The drawing under review shows one solid part. Ordinate dimensions are in mm from its lowest x, y, z. A direction names the side the tool comes from. Round coordinates to 2 decimals unless told otherwise and drop trailing zeros. Order: outer loops, then holes, each group sorted by start corner. A loop starts at its lowest first (then second) coordinate and runs counter-clockwise, first axis right, second up.
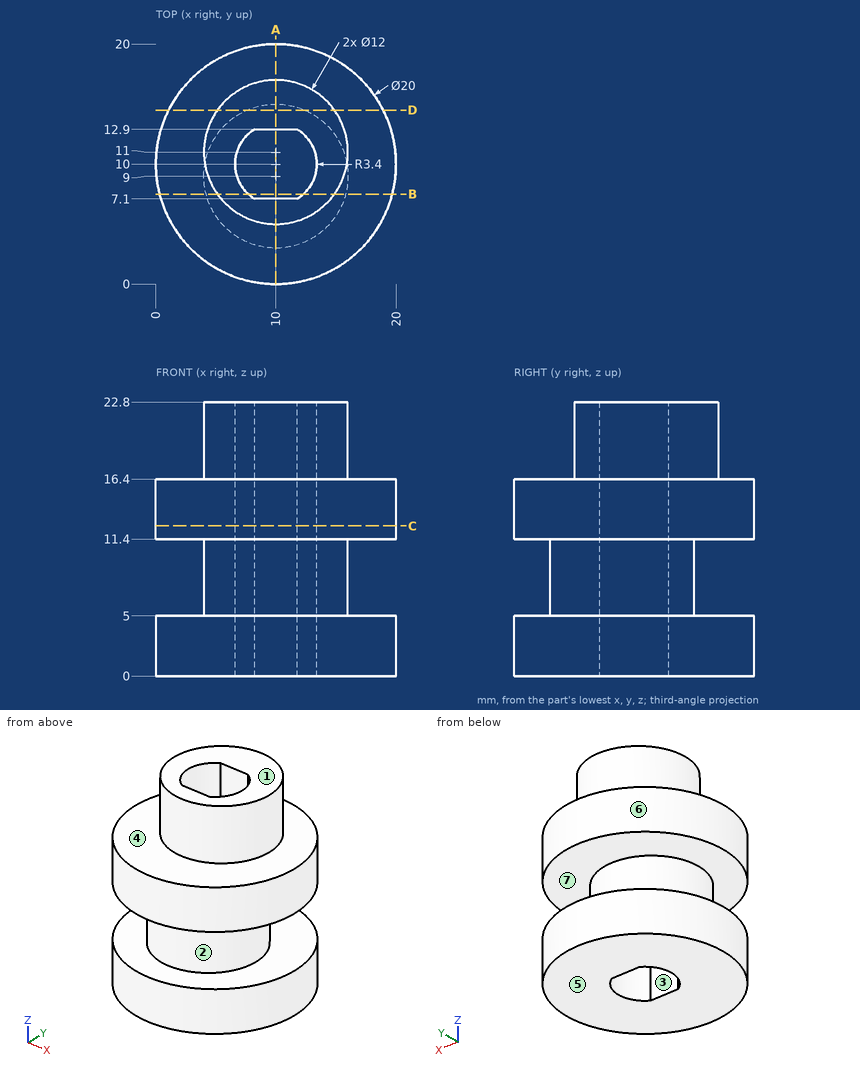
Q1. Tool access review of the marked faces 1, 2, 3 and 4: name each direction out of +Z, -Z, +X, -X, +Y, -Y from which nothing blocks a thin tool from reaching the whole face with its end or side.
Q2. Take a section at B-B, the plane y = 7.5. State the section outline as (x, z) points, plus the area to 3 significant figures.
Q3. Mouldability with a two-part tool opening along Z and no side actions: class the marked faces 5, 6 and 7 as +Z half, -Z half, draft (parallel to the pull), parting line (faces both ways), or undercut.
Q4. Take a section at C-C, the plane z = 12.5. State the section outline as (x, y) points.
Q5. Take a section at A-A, the plane x = 10. State the section outline as (y, z) points, plus the area to 3 significant figures.
Q6. Clearance check with flat-ended pins moving along their axes: pin 1 (1.5 mm diameter, centred on x = 8, y = 8.5, fed in from -Z); pin 2 (1.5 mm diameter, centred on x = 3.5, z = 15, fed in from +Y); pin 3 (1.5 mm diameter, centred on x = 17, y = 14.5, fed in from +Z); pin 4 (3 mm diameter, centred on x = 7, z = 7, fed in from +Y). State where each tip first meets the part, or that it passes through.
Q7. Take a section at D-D, the plane y = 14.5. State the section outline as (x, z) points.
Q8. Wall thickness on line 1 (Z direction, x = 5.5, y = 18.5); line 2 (X direction, y = 12.75, z = 6.75); line 3 (Y direction, x = 12.75, z = 6.75): over which ranges is each line inside the solid? List them lowest first.
Working result:
1. face 1: +Z, +X, -X, +Y, -Y
1. face 2: none
1. face 3: +Z, -Z
1. face 4: +Z
2. outline: (0.32, 0) - (7.7, 0) - (7.7, 22.8) - (5.13, 22.8) - (5.13, 16.4) - (0.32, 16.4) - (0.32, 11.4) - (4.19, 11.4) - (4.19, 5) - (0.32, 5) - close; (12.3, 0) - (19.68, 0) - (19.68, 5) - (15.81, 5) - (15.81, 11.4) - (19.68, 11.4) - (19.68, 16.4) - (14.87, 16.4) - (14.87, 22.8) - (12.3, 22.8) - close
2. area: 225 mm2
3. face 5: -Z half
3. face 6: draft
3. face 7: undercut
4. outline: circle Ø20 at (10, 10); hole (8.23, 7.1) - (11.77, 7.1) arc R3.4 ccw to (11.77, 12.9) - (8.23, 12.9) arc R3.4 ccw to start
5. outline: (0, 0) - (7.1, 0) - (7.1, 22.8) - (5, 22.8) - (5, 16.4) - (0, 16.4) - (0, 11.4) - (3, 11.4) - (3, 5) - (0, 5) - close; (12.9, 0) - (20, 0) - (20, 5) - (15, 5) - (15, 11.4) - (20, 11.4) - (20, 16.4) - (17, 16.4) - (17, 22.8) - (12.9, 22.8) - close
5. area: 221 mm2
6. pin 1: passes through
6. pin 2: stops at y = 18.18
6. pin 3: stops at z = 16.4
6. pin 4: stops at y = 14.81
7. outline: (1.07, 0) - (18.93, 0) - (18.93, 5) - (12.4, 5) - (12.4, 11.4) - (18.93, 11.4) - (18.93, 16.4) - (14.87, 16.4) - (14.87, 22.8) - (5.13, 22.8) - (5.13, 16.4) - (1.07, 16.4) - (1.07, 11.4) - (7.6, 11.4) - (7.6, 5) - (1.07, 5) - close
8. line 1: z = 0 to 5, 11.4 to 16.4
8. line 2: x = 5.32 to 8, 12 to 14.68
8. line 3: y = 3.67 to 8, 12 to 14.33
